from build123d import *

# Parameters (mm, degrees)
BOSS_EXTRUDE1_DEPTH = 18
SKETCH2_R           = 3.0000000000000004
SKETCH2_R_2         = 3.0000000000000013
BOSS_EXTRUDE3_DEPTH = 2
FILLET1_R           = 1
SKETCH3_R           = 2.250000000000001
CUT_EXTRUDE1_DEPTH  = 2
FILLET3_R           = 1


with BuildPart() as part:
    # Sketch1 → Boss-Extrude1 (new body)
    with BuildSketch(Plane.XY):
        Polygon((-50, 27), (0, 27.000000000000007), (0, 0), (-49.999999999999986, 0), align=None)
    extrude(amount=BOSS_EXTRUDE1_DEPTH)

    # Sketch2 → Boss-Extrude3 (add)
    with BuildSketch(Plane.ZY.offset(49.999999999999986)):
        with Locations(Location((9, 20.250000000000025, 0), (0, 0, 90))):
            Circle(SKETCH2_R)
        with Locations(Location((9, 6.749999999999998, 0), (0, 0, 90))):
            Circle(SKETCH2_R_2)
    extrude(amount=BOSS_EXTRUDE3_DEPTH)

    # Fillet1
    fillet1_edges = [part.edges().sort_by_distance(p)[0] for p in [
        (-51.99999999999999, 17.249999999999996, 9),
    ]]
    fillet(fillet1_edges, radius=FILLET1_R)

    # Sketch3 → Cut-Extrude1 (cut)
    with BuildSketch(Plane.ZY.offset(51.99999999999999)):
        with Locations(Location((9, 6.749999999999998, 0), (0, 0, 270))):
            Circle(SKETCH3_R)
    extrude(amount=-CUT_EXTRUDE1_DEPTH, mode=Mode.SUBTRACT)

    # Fillet3
    # the kernel refuses this fillet: 1 mm, written as the material it takes off along each edge
    with BuildSketch(Plane(origin=(-51.99999999999999, 6.749999999999972, 9), x_dir=(0, -1, 0), z_dir=(0, 0, -1))) as fillet3_piece_1:
        with BuildLine():
            CenterArc((3.25, -0.9682458365518585), FILLET3_R, 104.47751218592994, 75.52248781407006)
            Line((2.25, -0.9682458365518585), (2.2300000000000004, -0.9682458365518585))
            Line((2.2300000000000004, -0.9682458365518585), (2.2300000000000013, 0))
            Line((2.2300000000000013, 0), (2.250000000000001, 0.02000000000000313))
            ThreePointArc((2.250000000000001, 0.02000000000000313), (2.625000000000001, 0.01999999999999602), (2.9950000000000006, 0.01936491673102836))
            Line((2.9950000000000006, 0.01936491673102836), (3.0000000000000004, -7.11e-15))
        make_face()
    revolve(axis=Axis((-51.99999999999999, 6.749999999999972, 9), (-1, -5.1e-16, 0)), mode=Mode.SUBTRACT)


solid = part.part
Read the model definition and answer for the solid it produces. Units are mm, in the model's axes. A direction names the side the tool comes from. Coordinates: 2 decimals unless noted, no trailing zeros. Loops run counter-clockwise (first coordinate to the right, second up) from the corner with the lowest first, then second, coordinate; pieces in that order, holes last.
Q1. The part is cut by section C-C on z = 4.75. Write down the section's boundary in (x, y), and give its area (3 significant figures).
Q2. Consider probe 1 along Z at (x, y) = (-50.3, 6.75); probe 2 along X at (y, z) = (13.5, 1). Determine where each line is inside the solid, lowest interval first.
Q3. Each of these flat-tipped pins is pushed along its axis until it touches: pin 1 Ø5 at (y, z) = (5.5, 8.5) entering from -X; pin 2 Ø3 at (y, z) = (24, 15.5) entering from -X. Where does it stop, or does it pass through?
Q4. The part is cut by section A-A on z = 9. Write down the section's boundary in (x, y).
Q5. The part is cut by section B-B on y = 13.25. Write down the section's boundary in (x, z).
Q6. Which of the six approach directions +Z, -Z, +X, -X, +Y, -Y give full straight-line access (tool end or side, diameter ignored) to faces 1 (the face through (-50.52, 7.04, 11.23)), 2 (the face through (-25, 0, 9))?
Results below:
1. outline: (-50, 0) - (0, 0) - (0, 27) - (-50, 27) - close
1. area: 1,350 mm2
2. probe 1: z = 6 to 6.75, 11.25 to 12
2. probe 2: x = -50 to 0
3. pin 1: stops at x = -52
3. pin 2: stops at x = -50
4. outline: (-52, 3.75) - (-50, 3.75) - (-50, 0) - (0, 0) - (0, 27) - (-50, 27) - (-50, 23.25) - (-51, 23.25) arc R1 ccw to (-52, 22.25) - (-52, 18.25) arc R1 ccw to (-51, 17.25) - (-50, 17.25) - (-50, 9.75) - (-52, 9.75) arc R1 ccw to (-51.03, 9) - (-50, 9) - (-50, 4.5) - (-51.03, 4.5) arc R1 ccw to start
5. outline: (-50, 0) - (0, 0) - (0, 18) - (-50, 18) - close
6. face 1: -X
6. face 2: +Z, -Z, +X, -X, -Y
